from build123d import *

# Parameters (mm, degrees)
EXTRUDE_1_DEPTH     = 3
SKETCH_2_R          = 1.5
CUT_EXTRUDE_1_DEPTH = 3
SKETCH_3_R          = 1.5
SKETCH_3_R_2        = 25
SKETCH_3_R_3        = 15
SKETCH_3_R_4        = 2
CUT_EXTRUDE_2_DEPTH = 10
SKETCH_4_W          = 100
SKETCH_4_H          = 80
CUT_EXTRUDE_3_DEPTH = 3
FILLET_2_R          = 3
SKETCH_5_R          = 1.5
CUT_EXTRUDE_4_DEPTH = 3
FILLET_3_R          = 6
CHAMFER_1_SIZE      = 25
SKETCH_7_R          = 1.5
CUT_EXTRUDE_6_DEPTH = 10


with BuildPart() as part:
    # 草图1 → 凸台-拉伸1 (new body)
    with BuildSketch(Plane(origin=(0, 0, 0), x_dir=(1, 0, 0), z_dir=(0, 1, 0))):
        Polygon((-70, -53), (-70, -105), (70, -105), (70, -53), (140, -53), (140, 53), (70, 53), (70, 105), (-70, 105), (-70, 53), (-140, 53), (-140, -53), align=None)
    extrude(amount=EXTRUDE_1_DEPTH)

    # 草图2 → 切除-拉伸1 (cut)
    with BuildSketch(Plane(origin=(0, 3, 0), x_dir=(1, 0, 0), z_dir=(0, 1, 0))):
        with Locations(Location((120, 44, 0), (0, 0, 270))):
            Circle(SKETCH_2_R)
        with Locations(Location((90, 44, 0), (0, 0, 270))):
            Circle(SKETCH_2_R)
        with Locations(Location((90, 20, 0), (0, 0, 270))):
            Circle(SKETCH_2_R)
        with Locations(Location((120, 20, 0), (0, 0, 270))):
            Circle(SKETCH_2_R)
        with Locations(Location((120, -20, 0), (0, 0, 90))):
            Circle(SKETCH_2_R)
        with Locations(Location((120, -44, 0), (0, 0, 90))):
            Circle(SKETCH_2_R)
        with Locations(Location((90, -20, 0), (0, 0, 90))):
            Circle(SKETCH_2_R)
        with Locations(Location((90, -44, 0), (0, 0, 90))):
            Circle(SKETCH_2_R)
        with Locations(Location((-90, -44, 0), (0, 0, 270))):
            Circle(SKETCH_2_R)
        with Locations(Location((-90, -20, 0), (0, 0, 270))):
            Circle(SKETCH_2_R)
        with Locations(Location((-120, -44, 0), (0, 0, 270))):
            Circle(SKETCH_2_R)
        with Locations(Location((-120, -20, 0), (0, 0, 270))):
            Circle(SKETCH_2_R)
        with Locations(Location((-120, 20, 0), (0, 0, 90))):
            Circle(SKETCH_2_R)
        with Locations(Location((-90, 20, 0), (0, 0, 90))):
            Circle(SKETCH_2_R)
        with Locations(Location((-90, 44, 0), (0, 0, 90))):
            Circle(SKETCH_2_R)
        with Locations(Location((-120, 44, 0), (0, 0, 90))):
            Circle(SKETCH_2_R)
    extrude(amount=-CUT_EXTRUDE_1_DEPTH, mode=Mode.SUBTRACT)

    # 草图3 → 切除-拉伸2 (cut)
    with BuildSketch(Plane(origin=(0, 3, 0), x_dir=(1, 0, 0), z_dir=(0, 1, 0))):
        with Locations(Location((-64.5, 87, 0), (0, 0, 270))):
            Circle(SKETCH_3_R)
        with Locations(Location((-64.5, 67, 0), (0, 0, 270))):
            Circle(SKETCH_3_R)
        with Locations(Location((0, 77, 0), (0, 0, 270))):
            Circle(SKETCH_3_R_2)
        with Locations(Location((34.2, -70, 0), (0, 0, 270))):
            Circle(SKETCH_3_R)
        with Locations(Location((34.2, -86, 0), (0, 0, 270))):
            Circle(SKETCH_3_R)
        with Locations(Location((0, -78, 0), (0, 0, 270))):
            Circle(SKETCH_3_R_3)
        with Locations(Location((-50, 85, 0), (0, 0, 270))):
            Circle(SKETCH_3_R_4)
        with Locations(Location((-50, 69, 0), (0, 0, 270))):
            Circle(SKETCH_3_R_4)
        with Locations(Location((50, 85, 0), (0, 0, 270))):
            Circle(SKETCH_3_R_4)
        with Locations(Location((50, 69, 0), (0, 0, 270))):
            Circle(SKETCH_3_R_4)
        with Locations(Location((38.5, 87, 0), (0, 0, 270))):
            Circle(SKETCH_3_R)
        with Locations(Location((38.5, 67, 0), (0, 0, 270))):
            Circle(SKETCH_3_R)
        with Locations(Location((-53.8, -86, 0), (0, 0, 270))):
            Circle(SKETCH_3_R)
        with Locations(Location((-53.8, -70, 0), (0, 0, 270))):
            Circle(SKETCH_3_R)
    extrude(amount=-CUT_EXTRUDE_2_DEPTH, mode=Mode.SUBTRACT)

    # 草图4 → 切除-拉伸3 (cut)
    with BuildSketch(Plane(origin=(0, 3, 0), x_dir=(1, 0, 0), z_dir=(0, 1, 0))):
        Rectangle(SKETCH_4_W, SKETCH_4_H)
    extrude(amount=-CUT_EXTRUDE_3_DEPTH, mode=Mode.SUBTRACT)

    # 圆角2
    fillet_2_edges = [part.edges().sort_by_distance(p)[0] for p in [
        (50, 1.5, -40),
        (50, 1.5, 40),
        (-50, 1.5, 40),
        (-50, 1.5, -40),
    ]]
    fillet(fillet_2_edges, radius=FILLET_2_R)

    # 草图5 → 切除-拉伸4 (cut)
    with BuildSketch(Plane(origin=(0, 3, 0), x_dir=(1, 0, 0), z_dir=(0, 1, 0))):
        with Locations(Location((-60, 50, 0), (0, 0, 270))):
            Circle(SKETCH_5_R)
        with Locations(Location((-45, 98, 0), (0, 0, 270))):
            Circle(SKETCH_5_R)
        with Locations(Location((60, 50, 0), (0, 0, 90))):
            Circle(SKETCH_5_R)
        with Locations(Location((45, 98, 0), (0, 0, 90))):
            Circle(SKETCH_5_R)
        with Locations(Location((45, -98, 0), (0, 0, 270))):
            Circle(SKETCH_5_R)
        with Locations(Location((60, -50, 0), (0, 0, 270))):
            Circle(SKETCH_5_R)
        with Locations(Location((-45, -98, 0), (0, 0, 90))):
            Circle(SKETCH_5_R)
        with Locations(Location((-60, -50, 0), (0, 0, 90))):
            Circle(SKETCH_5_R)
    extrude(amount=-CUT_EXTRUDE_4_DEPTH, mode=Mode.SUBTRACT)

    # 圆角3
    fillet_3_edges = [part.edges().sort_by_distance(p)[0] for p in [
        (-140, 1.5, 53),
        (-140, 1.5, -53),
        (-70, 1.5, -105),
        (70, 1.5, -105),
        (140, 1.5, -53),
        (140, 1.5, 53),
        (70, 1.5, 105),
        (-70, 1.5, 105),
    ]]
    fillet(fillet_3_edges, radius=FILLET_3_R)

    # 倒角1
    chamfer_1_edges = [part.edges().sort_by_distance(p)[0] for p in [
        (-70, 1.5, 53),
        (-70, 1.5, -53),
        (70, 1.5, -53),
        (70, 1.5, 53),
    ]]
    chamfer(chamfer_1_edges, length=CHAMFER_1_SIZE)

    # 草图7 → 切除-拉伸6 (cut)
    with BuildSketch(Plane(origin=(0, 3, 0), x_dir=(1, 0, 0), z_dir=(0, 1, 0))):
        with Locations(Location((-135, 30, 0), (0, 0, 270))):
            Circle(SKETCH_7_R)
        with Locations(Location((-85, 30, 0), (0, 0, 270))):
            Circle(SKETCH_7_R)
        with Locations(Location((-85, -30, 0), (0, 0, 270))):
            Circle(SKETCH_7_R)
        with Locations(Location((-135, -30, 0), (0, 0, 270))):
            Circle(SKETCH_7_R)
        with BuildLine():
            Line((-134, -15), (-134, 15))
            ThreePointArc((-134, 15), (-130, 19), (-126, 15))
            Line((-126, 15), (-126, -15))
            ThreePointArc((-126, -15), (-130, -19), (-134, -15))
        make_face()
        with BuildLine():
            Line((-70, -25), (-70, 25))
            ThreePointArc((-70, 25), (-65, 30), (-60, 25))
            Line((-60, 25), (-60, -25))
            ThreePointArc((-60, -25), (-65, -30), (-70, -25))
        make_face()
        with BuildLine():
            Line((-83.192388155, 49.878679656), (-71.878679656, 61.192388155))
            ThreePointArc((-71.878679656, 61.192388155), (-64.807611845, 61.192388155), (-64.807611845, 54.121320344))
            Line((-64.807611845, 54.121320344), (-76.121320344, 42.807611845))
            ThreePointArc((-76.121320344, 42.807611845), (-83.192388155, 42.807611845), (-83.192388155, 49.878679656))
        make_face()
        with BuildLine():
            Line((134, -15), (134, 15))
            ThreePointArc((134, 15), (130, 19), (126, 15))
            Line((126, 15), (126, -15))
            ThreePointArc((126, -15), (130, -19), (134, -15))
        make_face()
        with BuildLine():
            Line((70, -25), (70, 25))
            ThreePointArc((70, 25), (65, 30), (60, 25))
            Line((60, 25), (60, -25))
            ThreePointArc((60, -25), (65, -30), (70, -25))
        make_face()
    extrude(amount=-CUT_EXTRUDE_6_DEPTH, mode=Mode.SUBTRACT)


solid = part.part
Design review of the part built by this model. Coordinates are the model's own, in mm. Give positions to 0.01 mm unless a question says otherwise; leave off trailing zeros. Loops run counter-clockwise (first coordinate to the right, second up) from the corner with the lowest first, then second, coordinate; pieces in that order, holes last. Notation, with made-up numbers: (45.5, 3.5) - (56.5, 3.5) arc R18 ccw to (56.5, 28.5) - close; hole circle Ø9 at (4, 70). An arc over 180 degrees is marked (long way). Write item = value, one per line.
1) Take a section at C-C on y = 1.1. Count the separate pieces of the cut face and the enclosed holes in it, and give its area (3 significant figures).
Result sheet:
separate_pieces = 1
enclosed_holes = 48
area = 32,500 mm2
2) Take a section at A-A on z = 9.5. State the section outline as (x, y) points.
Result sheet:
outline = (-140, 0) - (-134, 0) - (-134, 3) - (-140, 3) - close; (-126, 0) - (-70, 0) - (-70, 3) - (-126, 3) - close; (-60, 0) - (-50, 0) - (-50, 3) - (-60, 3) - close; (50, 0) - (60, 0) - (60, 3) - (50, 3) - close; (70, 0) - (126, 0) - (126, 3) - (70, 3) - close; (134, 0) - (140, 0) - (140, 3) - (134, 3) - close
3) Take a section at D-D on x = 111.5. State the section outline as (y, z) points.
Result sheet:
outline = (0, -53) - (3, -53) - (3, 53) - (0, 53) - close
4) Draft analysis for pull direction X (two halves, no side actions). For faces 1 (the face through (-2, 0, -48)), 2 (the face through (-77.61, 1.52, -55.46)), 3 (the face through (83, 1, 65)), 4 (the face through (-138.196, 1.521, 51.289)), state which applies: +X half, -X half, draft (parallel to the pull), parting line (faces both ways), or undercut.
Result sheet:
face_1 = draft
face_2 = undercut
face_3 = +X half
face_4 = -X half
5) Take a section at B-B on x = 4. State the section outline as (y, z) points.
Result sheet:
outline = (0, -105) - (3, -105) - (3, -101.68) - (0, -101.68) - close; (0, -52.32) - (3, -52.32) - (3, -40) - (0, -40) - close; (0, 40) - (3, 40) - (3, 63.54) - (0, 63.54) - close; (0, 92.46) - (3, 92.46) - (3, 105) - (0, 105) - close
6) To check wall thickness, follow line 1 (X direction, y = 1.9, z = 14); line 2 (X direction, y = 0.7, z = 44); line 3 (X direction, y = 2.45, z = 50). State the ranges of each line that lie inside material, in increasing order.
Result sheet:
line_1 = -140 to -134, -126 to -70, -60 to -50, 50 to 60, 70 to 126, 134 to 140
line_2 = -140 to -121.5, -118.5 to -91.5, -88.5 to 88.5, 91.5 to 118.5, 121.5 to 140
line_3 = -139.2 to -61.5, -58.5 to 58.5, 61.5 to 139.2
